Could you check a few things on this drawing? It's one solid part, dimensions in mm from its lowest x, y, z. Coordinates: 2 decimals unless noted, no trailing zeros. Loops run counter-clockwise (first coordinate to the right, second up) from the corner with the lowest first, then second, coordinate; pieces in that order, holes last.
1) If I drill on line 1 along Y through (x, z) = (6.25, 7.75); line 2 along Z through (x, y) = (3.5, 6.5); line 3 along Z through (x, y) = (7, 7.25) (1 decimal), over which ranges is the centre line in solid material (lowest first)?
2) Will these pins go through, and if not, where does the flat tip stop? P1, Ø1, axis at x = 3, y = 5, coming from the -Z side; P2, Ø3, axis at x = 3, z = 3, coming from the -Y side; P3, Ø1, axis at x = 1.5, y = 3, coming from the +Z side (1 decimal).
3) Thinking about a two-plate mould opening in Z: for the marked faces 1, 2 and 3, which applies, released by +Z, released by -Z, zero draft, split by the parting line, or undercut?
4) Imagine slicing it at A-A on z = 6. Please give me the cut outline in (x, y) (1 decimal), plus the area to 3 significant figures.
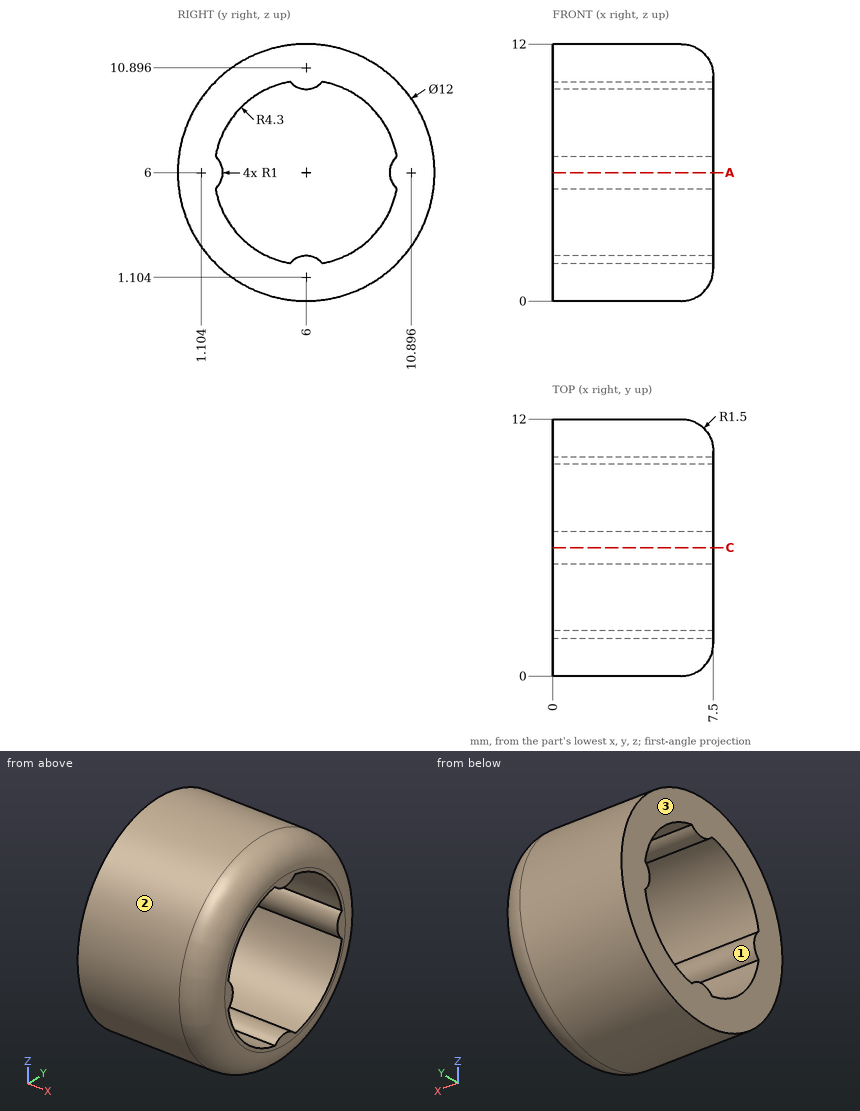
Filled in:
1. line 1: y = 0.28 to 2.07, 9.93 to 11.72
1. line 2: z = 0.02 to 1.97, 10.03 to 11.98
1. line 3: z = 0.5 to 1.9, 10.1 to 11.5
2. P1: stops at z = 0.02
2. P2: stops at y = 0.19
2. P3: stops at z = 11.5
3. face 1: undercut
3. face 2: split by the parting line
3. face 3: zero draft
4. outline: (0, 0) - (6, 0) arc R1.5 ccw to (7.5, 1.5) - (7.5, 2.1) - (0, 2.1) - close; (0, 9.9) - (7.5, 9.9) - (7.5, 10.5) arc R1.5 ccw to (6, 12) - (0, 12) - close
4. area: 30.6 mm2
